Work out the finished part from the listing and answer in its coordinate system (mm). A direction names the side the tool comes from. Coordinates: 2 decimals unless noted, no trailing zeros. Loops run counter-clockwise (first coordinate to the right, second up) from the corner with the lowest first, then second, coordinate; pieces in that order, holes last. Notation, with made-up numbers: (44.5, 46) -> (65.5, 46) arc R20 ccw to (65.5, 75) -> close; hole circle Ø2 at (2, -1.5). An arc over 180 degrees is marked (long way). Use a Markdown table: item, result.
from build123d import *

# Parameters (mm, degrees)
FILLET1_R = 1.524


with BuildPart() as part:
    # Sketch1 → Revolve1 (revolve)
    with BuildSketch(Plane(origin=(0, 0, 0), x_dir=(1, 0, 0), z_dir=(0, 1, 0))):
        Polygon((-37.029204897, 17.4625), (-37.029204897, 19.05), (-24.329204897, 19.05), (-17.145, 27.94), (3.175, 27.94), (3.175, 0), (0, 0), (0, 24.765), (-15.628644606, 24.765), (-22.812849503, 15.875), (-35.429004897, 15.875), (-35.429004897, 17.4625), align=None)
    revolve(axis=Axis((3.175, 0, 0), (-1, 0, 0)))

    # Fillet1
    fillet1_edges = [part.edges().sort_by_distance(p)[0] for p in [
        (3.175, 0, 27.94),
        (-17.145, 0, 27.94),
    ]]
    fillet(fillet1_edges, radius=FILLET1_R)


solid = part.part
Q1. For faces 1 (the cylindrical face through (-7.26, -27.7, 3.64)), 2 (the cylindrical face through (-29.209, 15.497, 3.441)), 3 (the conical face through (-22.464, 14.467, -7.525)), determine the directions among +Z, -Z, +X, -X, +Y, -Y from which every point of the face is accessible in a straight line to the end or side of a thin tool.
Solved:
| item | result |
|---|---|
| face 1 | +X, -X |
| face 2 | -X |
| face 3 | none |
Q2. Given pin 1 Ø12 at (x, y) = (-18, -8.5) entering from -Z; pin 2 Ø1 at (x, z) = (-31, -2) entering from +Y, each flat-ended and moving along its own axis, determine where each tip first touches the part or whether it passes through.
Solved:
| item | result |
|---|---|
| pin 1 | z = -27.81 |
| pin 2 | y = 18.99 |
Q3. Determine the mould class of faces 4 (the conical face through (-23.908, -5.879, -18.667)), 5 (the cylindrical face through (-7.92, -7.44, -23.62)), 6 (the cylindrical face through (-36.24, 10.626, 13.858)) for opening direction X: pulls with the +X half, pulls with the -X half, needs draft (parallel to the pull), parting line crosses it, or undercut.
Solved:
| item | result |
|---|---|
| face 4 | pulls with the -X half |
| face 5 | undercut |
| face 6 | needs draft |
Q4. Consider line 1 (Y direction, x = -27.5, z = 0) (3 decimals); line 2 (Z direction, x = -36.4, y = 0). Determine where each line is inside the solid, lowest interval first. Write a range as [from, to].
Solved:
| item | result |
|---|---|
| line 1 | [-19.05, -15.875], [15.875, 19.05] |
| line 2 | [-19.05, -17.46], [17.46, 19.05] |
Q5. Section A-A on x = -3 is taken. Determine the outline of the cut face in (y, z) (3 decimals).
Solved:
| item | result |
|---|---|
| outline | circle Ø55.88 at (0, 0); hole circle Ø49.53 at (0, 0) |
Q6. Section B-B on x = -30 is taken. Determine the outline of the cut face in (y, z) (3 decimals).
Solved:
| item | result |
|---|---|
| outline | circle Ø38.1 at (0, 0); hole circle Ø31.75 at (0, 0) |
